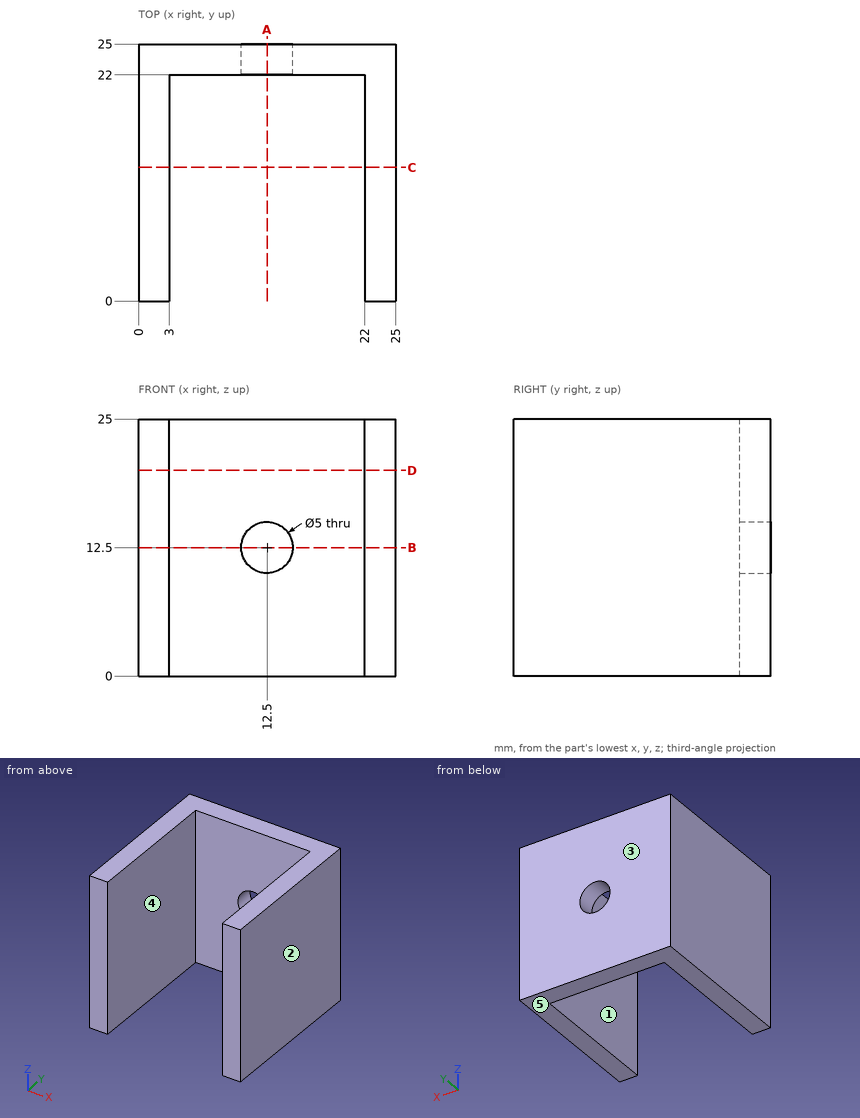
Design review of the part shown in the three views and the two pictorial views. Dimensions are in mm from the part's minimum x, y and z. A direction names the side the tool comes from. Round coordinates to 2 decimals unless told otherwise and drop trailing zeros. Order: outer loops, then holes, each group sorted by start corner. A loop starts at its lowest first (then second) coordinate and runs counter-clockwise, first axis right, second up. Notation, with made-up numbers: (82.5, -17) - (122.5, -17) arc R36 ccw to (122.5, 20) - close; hole circle Ø4 at (9, 31.25). An arc over 180 degrees is marked (long way). Answer in a Markdown table with one row per item.
(1) Take a section at A-A on x = 12.5. Write out the cut boundary in (y, z), plus the area to 3 significant figures.
Result set:
| item | result |
|---|---|
| outline | (22, 0) - (25, 0) - (25, 10) - (22, 10) - close; (22, 15) - (25, 15) - (25, 25) - (22, 25) - close |
| area | 60.0 mm2 |
(2) Mouldability with a two-part tool opening along X and no side actions: class the marked faces 1, 2 and 3 as released by +X, released by -X, zero draft, split by the parting line, or undercut.
Result set:
| item | result |
|---|---|
| face 1 | undercut |
| face 2 | released by +X |
| face 3 | zero draft |
(3) Machinability: for the marked faces 4 and 5, which of the approach directions +Z, -Z, +X, -X, +Y, -Y give a long, thin tool a straight path to every point of the face, cutting with its end or side? Answer none if there is none.
Result set:
| item | result |
|---|---|
| face 4 | +Z, -Z, -Y |
| face 5 | -Z, +X, -X, +Y, -Y |
(4) Take a section at C-C on y = 13. Write out the cut boundary in (x, z).
Result set:
| item | result |
|---|---|
| outline | (0, 0) - (3, 0) - (3, 25) - (0, 25) - close; (22, 0) - (25, 0) - (25, 25) - (22, 25) - close |
(5) For line 1 (X direction, y = 7.5, z = 22.5); line 2 (Z direction, x = 12.5, y = 23.8); line 3 (Y direction, x = 13, z = 1.5), list the stretches that pass through material, from the lowest coordinate up. Write a range as from..to.
Result set:
| item | result |
|---|---|
| line 1 | x = 0..3, 22..25 |
| line 2 | z = 0..10, 15..25 |
| line 3 | y = 22..25 |
(6) Take a section at B-B on z = 12.5. Write out the cut boundary in (x, y), plus the area to 3 significant figures.
Result set:
| item | result |
|---|---|
| outline | (0, 0) - (3, 0) - (3, 22) - (10, 22) - (10, 25) - (0, 25) - close; (15, 22) - (22, 22) - (22, 0) - (25, 0) - (25, 25) - (15, 25) - close |
| area | 192 mm2 |
(7) Take a section at D-D on z = 20. Write out the cut boundary in (x, y).
Result set:
| item | result |
|---|---|
| outline | (0, 0) - (3, 0) - (3, 22) - (22, 22) - (22, 0) - (25, 0) - (25, 25) - (0, 25) - close |
(8) Clearance check with flat-ended pins moving along their axes: P1, Ø3, axis at x = 12.5, z = 12.5, coming from the -Y side; P2, Ø8, axis at x = 11.5, z = 13.5, coming from the -Y side. State where each tip first meets the part, or that it passes through.
Result set:
| item | result |
|---|---|
| P1 | passes through |
| P2 | stops at y = 22 |
